Autodesk Inventor part; units mm, degrees
ref_plane "YZ Plane" through (0, 0, 0) normal (1, 0, 0) x (0, 1, 0)
ref_plane "XZ Plane" through (0, 0, 0) normal (0, 1, 0) x (-1, 0, 0)
ref_plane "XY Plane" through (0, 0, 0) normal (0, 0, 1) x (1, 0, 0)
sketch "Sketch1" plane through (0, 0, 0) normal (0, 0, 1) x (1, 0, 0)
  line L0 (-144, -30) -> (144, -30)
  line L1 (144, -30) -> (144, 30)
  line L2 (144, 30) -> (-144, 30)
  line L3 (-144, 30) -> (-144, -30)
  line L4 (-144, -30) -> (144, 30) construction
  line L5 (144, -30) -> (-144, 30) construction
  line L6 (144, 30) -> (101.9875, -30)
  line L7 (-144, 30) -> (-101.9875, -30)
  point P0 (0, 0)
  dimension "d0" = 288
  dimension "d1" = 60
  dimension "d2" = 55
  dimension "d13" = 55
extrude "Extrusion1" add sketch "Sketch1" along normal blind 3 contours L7 L2 L6 L0
sketch "Sketch2" plane through (0, 0, 3) normal (0, 0, 1) x (1, 0, 0)
  circle A0 centre (-100, -5) radius 1.65
  line L0 (-101.9875, -30) -> (101.9875, -30)
  line L1 (-100, -5) -> (155.6099, -5) construction
  circle A1 centre (100, -5) radius 1.65
  point P0 (0, 0)
  dimension "d5" = 25
  dimension "d6" = 3.3
  dimension "d9" = 3.3
  dimension "d14" = 100
  dimension "d15" = 100
extrude "Extrusion2" cut sketch "Sketch2" against normal through all
fillet "Fillet1" radius 2 3 edges at (-144, 30, 1.5) (101.9875, -30, 1.5) (144, 30, 1.5)
sketch "Sketch3" plane through (0, 0, 3) normal (0, 0, 1) x (1, 0, 0)
  arc A0 (141.7963, 26.8528) -> (140.158, 30) centre (140.158, 28) ccw
  line L0 (140.158, 30) -> (-140.158, 30)
  arc A1 (-140.158, 30) -> (-141.7963, 26.8528) centre (-140.158, 28) ccw
  line L1 (-141.7963, 26.8528) -> (-101.9875, -30)
  line L2 (-101.9875, -30) -> (100.9464, -30)
  arc A2 (100.9464, -30) -> (102.5847, -29.1472) centre (100.9464, -28) ccw
  line L3 (102.5847, -29.1472) -> (141.7963, 26.8528)
  circle A3 centre (-100, -5) radius 1.65
  circle A4 centre (100, -5) radius 1.65
  point P0 (0, 0)
equation "\"d13\" = d2"
equation "\"d9\" = d6"
properties part number "UpperAcrylicSheetBack"
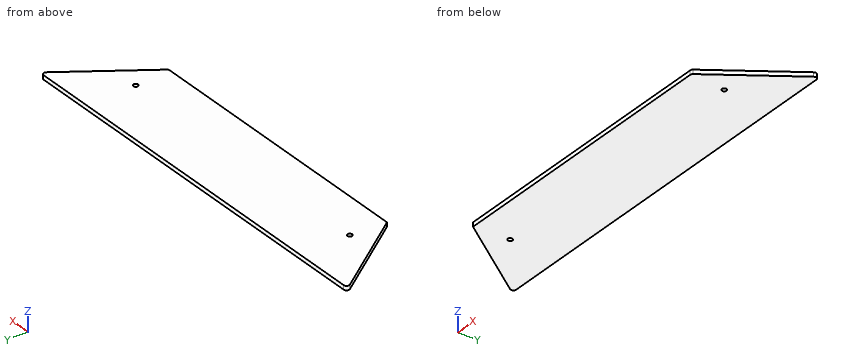
Design review of the part built by this model. Coordinates are the model's own, in mm. Coordinates: 2 decimals unless noted, no trailing zeros. Order: outer loops, then holes, each group sorted by start corner. A loop starts at its lowest first (then second) coordinate and runs counter-clockwise, first axis right, second up.
1) Wall thickness on line 1 along Y through (x, z) = (-100, 2.1); line 2 along X through (y, z) = (-6.5, 0.45); line 3 along X through (y, z) = (14.5, 2.6): over which ranges is each line inside the solid? List them lowest first.
2) Clearance check with a flat-ended pin moving along its axis: pin 1 (1.5 mm diameter, centred on y = -17, z = 2, fed in from -X). State where the tip first meets the part, or that it passes through.
3) Take a section at A-A, the plane z = 1.1. Give the boundary of the cut face in (x, y), and give its area (3 significant figures).
4) Take a section at B-B, the plane y = 16. Give the boundary of the cut face in (x, z).
5) Take a section at C-C, the plane x = -107.5. Give the boundary of the cut face in (y, z).
Returned:
1. line 1: y = -30 to -6.65, -3.35 to 30
1. line 2: x = -118.44 to -100.69, -99.31 to 99.31, 100.69 to 118.44
1. line 3: x = -133.15 to 133.15
2. pin 1: stops at x = -111.62
3. outline: (-141.8, 26.85) - (-101.99, -30) - (100.95, -30) arc R2 ccw to (102.58, -29.15) - (141.8, 26.85) arc R2 ccw to (140.16, 30) - (-140.16, 30) arc R2 ccw to start; hole circle Ø3.3 at (-100, -5); hole circle Ø3.3 at (100, -5)
3. area: 14,700 mm2
4. outline: (-134.2, 0) - (134.2, 0) - (134.2, 3) - (-134.2, 3) - close
5. outline: (-22.13, 0) - (30, 0) - (30, 3) - (-22.13, 3) - close
